For this review, use the dimensioned drawing (mm, ordinates from the lowest corner) and the shaded views. A direction names the side the tool comes from. Give positions to 0.01 mm unless a question says otherwise; leave off trailing zeros. Write each loop counter-clockwise with the first axis right and the second up, starting at its lowest first coordinate (ties: lowest second). Pieces come first, ordered by that corner, then holes.
1) We need section B-B on x = 27. Give the boundary of the cut face in (y, z), and give its area (3 significant figures).
2) Wall thickness on line 1 along Y through (x, z) = (56, 50.5); line 2 along Z through (x, y) = (60.5, 28.5); line 3 along X through (y, z) = (19, 49): over which ranges is each line inside the solid? List them lowest first.
3) Draft analysis for pull direction Z (two halves, no side actions). For the marked faces 1, 2 and 3, state which applies: pulls with the +Z half, pulls with the -Z half, needs draft (parallel to the pull), parting line crosses it, or undercut.
4) For P1, Ø10, axis at x = 60.5, z = 59.5, coming from the +Y side; P2, Ø16, axis at y = 44.5, z = 61, coming from the -X side; P3, Ø2, axis at y = 15, z = 9.5, coming from the +X side; P4, Ø11, axis at x = 25.5, y = 52, coming from the -Z side, all flat-tipped, find the tip position at first contact; note any pin that passes through.
5) Machinability: for the marked faces 4, 5 and 6, which of the approach directions +Z, -Z, +X, -X, +Y, -Y give a long, thin tool a straight path to every point of the face, cutting with its end or side? Answer none if there is none.
6) We need section D-D on x = 35.5. Give the boundary of the cut face in (y, z).
7) We need section C-C on y = 65.5. Give the boundary of the cut face in (x, z).
8) We need section A-A on z = 45.5. Give the boundary of the cut face in (x, y).
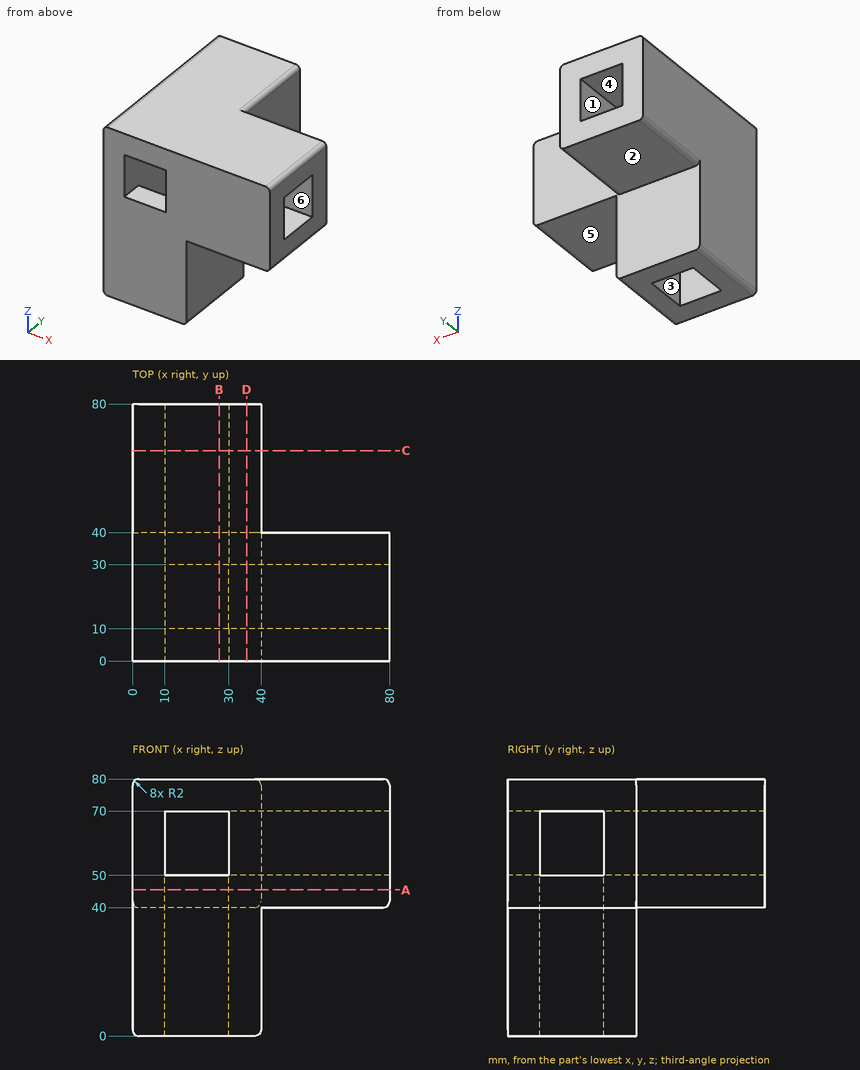
Results list:
1. outline: (0, 0) - (10, 0) - (10, 50) - (0, 50) - close; (0, 70) - (80, 70) - (80, 80) - (0, 80) - close; (30, 0) - (40, 0) - (40, 40) - (80, 40) - (80, 50) - (30, 50) - close
1. area: 2,200 mm2
2. line 1: y = 0 to 10, 30 to 40
2. line 2: z = 40 to 50, 70 to 80
2. line 3: x = 0 to 10, 30 to 80
3. face 1: undercut
3. face 2: pulls with the -Z half
3. face 3: needs draft
4. P1: stops at y = 40
4. P2: stops at x = 0
4. P3: stops at x = 40
4. P4: stops at z = 40
5. face 4: none
5. face 5: -Z, +X, +Y, -Y
5. face 6: +X
6. outline: (0, 0) - (40, 0) - (40, 40) - (80, 40) - (80, 80) - (0, 80) - close; hole (10, 50) - (30, 50) - (30, 70) - (10, 70) - close
7. outline: (0, 42) arc R2 ccw to (2, 40) - (38, 40) arc R2 ccw to (40, 42) - (40, 78) arc R2 ccw to (38, 80) - (2, 80) arc R2 ccw to (0, 78) - close; hole (10, 50) - (30, 50) - (30, 70) - (10, 70) - close
8. outline: (0, 0) - (80, 0) - (80, 40) - (40, 40) - (40, 80) - (0, 80) - close; hole (10, 10) - (30, 10) - (30, 30) - (10, 30) - close
